The listing builds one solid part. Answer for the finished solid, in the listing's coordinates (mm). Face numbers are marked on the shaded views. A direction names the side the tool comes from. Round coordinates to 2 decimals unless told otherwise and drop trailing zeros. Loops run counter-clockwise (first coordinate to the right, second up) from the corner with the lowest first, then second, coordinate; pieces in that order, holes last. Notation, with made-up numbers: M -12,12.5 L 31,12.5 A13 cw 31,28.5 Z; hole C 10,-14.75 d5. An arc over 180 degrees is marked long. Put each result on its own line as item: value. Start each with the question number.
(1) A flat-ended cylindrical pin translates along its axis: P1, Ø5, axis at x = -3.5, z = -3.5, coming from the +Y side. Find the tip coordinate at first contact, or state that the pin passes through.
(2) Straight lines are drawn through the part: line 1 (Z direction, x = -3.5, y = 0.85); line 2 (X direction, y = 1.3, z = -8.75); line 3 (Z direction, x = -78.5, y = 1.85). For each, find the intervals that lie inside material, in ascending order.
(3) Section C-C, the plane x = -96.5 is taken. Determine the outline of the cut face in (y, z).
(4) Section D-D, the plane x = -64.5 is taken. Determine the outline of the cut face in (y, z), then the cut area to 3 significant figures.
(5) Section B-B, the plane y = 2.25 is taken. Determine the outline of the cut face in (x, z).
(6) Section A-A, the plane z = -3.5 is taken. Determine the outline of the cut face in (x, y).
(7) Which of the six approach directions +Z, -Z, +X, -X, +Y, -Y give full straight-line access (tool end or side, diameter ignored) to the marked faces 1 and 2?
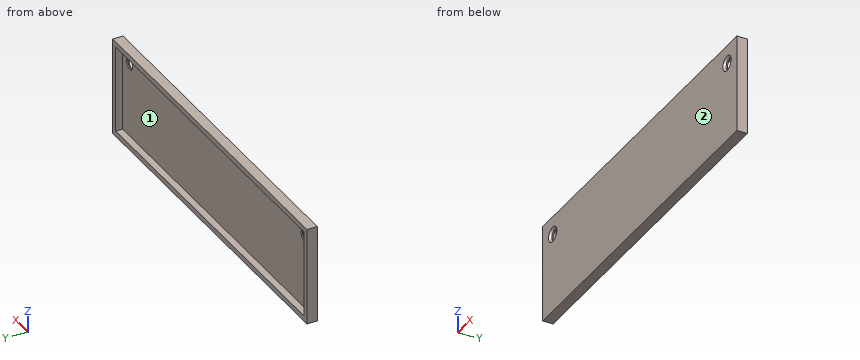
Autodesk Inventor part; units mm, degrees
ref_plane "YZ Plane" through (0, 0, 0) normal (1, 0, 0) x (0, 1, 0)
ref_plane "XZ Plane" through (0, 0, 0) normal (0, 1, 0) x (-1, 0, 0)
ref_plane "XY Plane" through (0, 0, 0) normal (0, 0, 1) x (1, 0, 0)
sketch "Szkic1" plane through (0, 0, 0) normal (0, 1, 0) x (-1, 0, 0)
  circle A0 centre (3.5, -3.5) radius 1.6
  circle A1 centre (96.5, -3.5) radius 1.6
  line L0 (100, 0) -> (100, -25)
  line L1 (100, -25) -> (0, -25)
  line L2 (0, -25) -> (0, 0)
  line L3 (0, 0) -> (100, 0)
  line L4 (100.2, -25.2) -> (100.2, 0.2)
  line L5 (100.2, 0.2) -> (-0.2, 0.2)
  line L6 (-0.2, 0.2) -> (-0.2, -25.2)
  line L7 (-0.2, -25.2) -> (100.2, -25.2)
  line L8 (101.8, -26.8) -> (101.8, 1.8)
  line L9 (101.8, 1.8) -> (-1.8, 1.8)
  line L10 (-1.8, 1.8) -> (-1.8, -26.8)
  line L11 (-1.8, -26.8) -> (101.8, -26.8)
  dimension "d0" = 0.2
  dimension "d1" = 1.6
extrude "Wyciągnięcie proste1" add sketch "Szkic1" along normal blind 1 contours L0 L1 L2 L3 | L7 L6 L5 L4 | L11 L10 L9 L8
extrude "Wyciągnięcie proste2" add sketch "Szkic1" along normal blind 3 contours L11 L10 L9 L8
chamfer "Faza1" distance 0.6 angle 45 2 edges at (-1.9, 0, -3.5) (-94.9, 0, -3.5)
properties part number "forma_noz"
Recorded:
1. P1: stops at y = 1
2. line 1: z = -26.8 to -5.1, -1.9 to 1.8
2. line 2: x = -101.8 to -100.2, 0.2 to 1.8
2. line 3: z = -26.8 to -25.2, 0.2 to 1.8
3. outline: M 0,-26.8 L 3,-26.8 L 3,-25.2 L 1,-25.2 L 1,-5.1 L 0.6,-5.1 L 0,-5.7 Z; M 0,-1.3 L 0.6,-1.9 L 1,-1.9 L 1,0.2 L 3,0.2 L 3,1.8 L 0,1.8 Z
4. outline: M 0,-26.8 L 3,-26.8 L 3,-25.2 L 1,-25.2 L 1,0.2 L 3,0.2 L 3,1.8 L 0,1.8 Z
4. area: 35.0 mm²
5. outline: M -101.8,-26.8 L 1.8,-26.8 L 1.8,1.8 L -101.8,1.8 Z; hole M -100.2,-25.2 L 0.2,-25.2 L 0.2,0.2 L -100.2,0.2 Z
6. outline: M -101.8,0 L -98.7,0 L -98.1,0.6 L -98.1,1 L -100.2,1 L -100.2,3 L -101.8,3 Z; M -94.9,0.6 L -94.3,0 L -5.7,0 L -5.1,0.6 L -5.1,1 L -94.9,1 Z; M -1.9,0.6 L -1.3,0 L 1.8,0 L 1.8,3 L 0.2,3 L 0.2,1 L -1.9,1 Z
7. face 1: +Y
7. face 2: +Z, -Z, +X, -X, -Y
